from build123d import *

# Parameters (mm, degrees)
F1_DEPTH = 10
F3_DEPTH = 10
F4_W     = 87
F4_H     = 11
F5_DEPTH = 10
F6_W     = 11
F6_H     = 50
F7_DEPTH = 10


with BuildPart() as f1:
    # F0 (on Top) → F1 (new body)
    with BuildSketch(Plane.XY):
        Polygon((150, 110), (-150, 110), (-150, -110), (-69, -110), (150, -110), align=None)
    extrude(amount=F1_DEPTH)

    # F2 (on face) → F3 (cut)
    with BuildSketch(Plane.XY.offset(10)):
        Polygon((140, 48), (140, 100), (85, 100), (85, 89), (129, 89), (129, 48), align=None)
        Polygon((-85, 100), (-140, 100), (-140, 48), (-129, 48), (-129, 89), (-85, 89), align=None)
        Polygon((-140, -48), (-140, -100), (-85, -100), (-85, -89), (-129, -89), (-129, -48), align=None)
        Polygon((85, -100), (140, -100), (140, -48), (129, -48), (129, -89), (85, -89), align=None)
    extrude(amount=-F3_DEPTH, mode=Mode.SUBTRACT)

    # F4 (on face) → F5 (cut)
    with BuildSketch(Plane.XY.offset(10)):
        with Locations((0, 94.5)):
            Rectangle(F4_W, F4_H)
        with Locations((0, -94.5)):
            Rectangle(F4_W, F4_H)
    extrude(amount=-F5_DEPTH, mode=Mode.SUBTRACT)

    # F6 (on face) → F7 (cut)
    with BuildSketch(Plane.XY.offset(10)):
        with Locations((-134.5, 0)):
            Rectangle(F6_W, F6_H)
        Polygon((140, -25), (140, 0), (140, 25), (129, 25), (129, -25), align=None)
    extrude(amount=-F7_DEPTH, mode=Mode.SUBTRACT)


solid = f1.part
Geometry: final body of the model. Coordinates: model frame, mm. Coordinates: 2 decimals unless noted, no trailing zeros. Order: outer loops, then holes, each group sorted by start corner. A loop starts at its lowest first (then second) coordinate and runs counter-clockwise, first axis right, second up.
1) Draft query along Y for faces 1 (the flat face through (-43.5, 94, 5)), 2 (the flat face through (2, 110, 5)), 3 (the flat face through (135, 25, 5)), 4 (the flat face through (-2, 2, 0)). Return one class per face: released by +Y, released by -Y, zero draft, split by the parting line, or undercut.
Result sheet:
face 1: undercut
face 2: released by +Y
face 3: undercut
face 4: zero draft
2) Section B-B (x = 40). Return loops of the section in (y, z), then the cut area to 3 significant figures.
Result sheet:
outline: (-110, 0) - (-100, 0) - (-100, 10) - (-110, 10) - close; (-89, 0) - (89, 0) - (89, 10) - (-89, 10) - close; (100, 0) - (110, 0) - (110, 10) - (100, 10) - close
area: 1,980 mm2
3) Section C-C (z = 5.25). Give the number of separate pieces and of enclosed holes in the cut face, then the cut area to 3 significant figures.
Result sheet:
separate pieces: 1
enclosed holes: 8
area: 58,800 mm2
4) Ray query, probe 1 along Y at (x, z) = (-43, 6.75); probe 2 along X at (y, z) = (15, 3). Return the intervals inside material, ascending.
Result sheet:
probe 1: y = -110 to -100, -89 to 89, 100 to 110
probe 2: x = -150 to -140, -129 to 129, 140 to 150
5) Section A-A (y = 15.5). Return loops of the section in (x, z).
Result sheet:
outline: (-150, 0) - (-140, 0) - (-140, 10) - (-150, 10) - close; (-129, 0) - (129, 0) - (129, 10) - (-129, 10) - close; (140, 0) - (150, 0) - (150, 10) - (140, 10) - close
